CAD build for the part. Positions are in the model's coordinates, mm. A direction names the side the tool comes from. Round coordinates to 2 decimals unless told otherwise and drop trailing zeros. Write each loop counter-clockwise with the first axis right and the second up, starting at its lowest first coordinate (ties: lowest second). Pieces come first, ordered by that corner, then holes. Notation, with made-up numbers: (65.25, 74.25) -> (74.25, 74.25) arc R32 cw to (74.25, 109.25) -> close; hole circle Ø3 at (-1, 26). An arc over 180 degrees is marked (long way). Put each result on its own line as item: value. Start each with the question number.
1. Drill centre lines: line 1 (Z direction, x = 33.9, y = 0); line 2 (Y direction, x = 35.8, z = 16); line 3 (Y direction, x = 34.5, z = 37.5). Where is each one in solid material? Low to high. Write a range as from..to.
2. 3-axis set-ups, long thin cutter, end or side, ignore diameter. For faces 4 (the flat face through (36, 2, 20)), 5 (the cylindrical face through (39.82, 5.56, 40.66)), 6 (the cylindrical face through (35.637, -0.432, 71.197)), 7 (the flat face through (37, 14, 41)): which of +Z, -Z, +X, -X, +Y, -Y reach the whole face in a straight line?
3. Saw through at C-C on z = 41.2. List the corners of the cut face in (x, y).
4. Saw through at A-A on z = 8. List the corners of the cut face in (x, y).
5. Flat gauge pins, fed straight in: P1, Ø3.5, axis at x = 36, y = -10.5, coming from the +Z side; P2, Ø8, axis at y = -8, z = 41.2, coming from the +X side; P3, Ø17.5, axis at y = 10.5, z = 13.5, coming from the +X side; P4, Ø1.4, axis at y = 11, z = 16, coming from the +X side. Where does each tip first touch, or does it go through?
6. Pull direction X, two halves, no side cores. Call faces 1 (the cylindrical face through (36.608, -10.399, -4.437)), 2 (the flat face through (39.2, 7, 42)), 3 (the flat face through (35, 11, -9)): pulls with the +X half, pulls with the -X half, needs draft (parallel to the pull), parting line crosses it, or undercut.
7. Saw through at D-D on y = 22.5. List the corners of the cut face in (x, z), and give its area (3 significant figures).
8. Saw through at B-B on z = 22. List the corners of the cut face in (x, y), and give its area (3 significant figures).
from build123d import *

# Parameters (mm, degrees)
SKETCH_1_W          = 9
SKETCH_1_H          = 60
EXTRUDE_1_DEPTH     = 41.2
SKETCH_4_R          = 30
EXTRUDE_3_DEPTH     = 9
CUT_EXTRUDE_1_DEPTH = 72
SKETCH_5_R          = 15.7
CUT_EXTRUDE_2_DEPTH = 3
SKETCH_6_W          = 4
SKETCH_6_H          = 28
CUT_EXTRUDE_3_DEPTH = 3
SKETCH_7_W          = 3
SKETCH_7_H          = 4
CUT_EXTRUDE_4_DEPTH = 39.2
SKETCH_8_W          = 4
SKETCH_8_H          = 82.4
CUT_EXTRUDE_5_DEPTH = 25
SKETCH_9_R          = 2
EXTRUDE_4_DEPTH     = 9
SKETCH_10_R         = 0.8
CUT_EXTRUDE_6_DEPTH = 5
SKETCH_11_R         = 1
CUT_EXTRUDE_7_DEPTH = 1
SKETCH_12_R         = 2.5
CUT_EXTRUDE_9_DEPTH = 2


with BuildPart() as part:
    # 草图1 → 凸台-拉伸1 (new body)
    with BuildSketch(Plane.XY):
        with Locations((36.7, 0)):
            Rectangle(SKETCH_1_W, SKETCH_1_H)
    extrude(amount=EXTRUDE_1_DEPTH)

    # 草图4 → 凸台-拉伸3 (add)
    with BuildSketch(Plane.ZY.offset(-32.2)):
        with Locations((41.2, 0)):
            Circle(SKETCH_4_R)
    extrude(amount=-EXTRUDE_3_DEPTH)

    # 切除-拉伸1: read off the stored shape, not the designer's step
    # 切除-拉伸1 outline → 切除-拉伸1 (cut)
    with BuildSketch(Plane.XY):
        with BuildLine():
            Line((32.2, 30), (32.2, 25.702139989))
            ThreePointArc((32.2, 25.702139989), (38.884958532, 13.616166862), (41.2, 0))
            Line((41.2, 0), (41.2, 30))
            Line((41.2, 30), (32.2, 30))
        make_face()
        with BuildLine():
            Line((41.2, -30), (41.2, 0))
            ThreePointArc((41.2, 0), (38.884958532, -13.616166862), (32.2, -25.702139989))
            Line((32.2, -25.702139989), (32.2, -30))
            Line((32.2, -30), (41.2, -30))
        make_face()
    extrude(amount=CUT_EXTRUDE_1_DEPTH, mode=Mode.SUBTRACT)

    # 草图5 → 切除-拉伸2 (cut)
    with BuildSketch(Plane.ZY.offset(-32.2)):
        with Locations((41.2, 0)):
            Circle(SKETCH_5_R)
    extrude(amount=-CUT_EXTRUDE_2_DEPTH, mode=Mode.SUBTRACT)

    # 草图6 → 切除-拉伸3 (cut)
    with BuildSketch(Plane.ZY.offset(-35.2)):
        with Locations((41.2, 0)):
            Rectangle(SKETCH_6_W, SKETCH_6_H)
    extrude(amount=-CUT_EXTRUDE_3_DEPTH, mode=Mode.SUBTRACT)

    # 草图7 → 切除-拉伸4 (cut)
    with BuildSketch(Plane.XY.offset(39.2)):
        with Locations((36.7, 0)):
            Rectangle(SKETCH_7_W, SKETCH_7_H)
    extrude(amount=-CUT_EXTRUDE_4_DEPTH, mode=Mode.SUBTRACT)

    # 草图8 → 切除-拉伸5 (cut)
    with BuildSketch(Plane.XY):
        with Locations((39.2, 0)):
            Rectangle(SKETCH_8_W, SKETCH_8_H)
    extrude(amount=CUT_EXTRUDE_5_DEPTH, mode=Mode.SUBTRACT)

    # 草图9 → 凸台-拉伸4 (add)
    with BuildSketch(Plane.XY):
        with Locations((34.7, 11)):
            Circle(SKETCH_9_R)
        with Locations((34.7, -11)):
            Circle(SKETCH_9_R)
    extrude(amount=-EXTRUDE_4_DEPTH)

    # 草图10 → 切除-拉伸6 (cut)
    with BuildSketch(Plane(origin=(37.2, 0, 0), x_dir=(0, 0, -1), z_dir=(1, 0, 0))):
        with Locations((-16, -11)):
            Circle(SKETCH_10_R)
        with Locations((-8, -11)):
            Circle(SKETCH_10_R)
        with Locations((-16, 11)):
            Circle(SKETCH_10_R)
        with Locations((-8, 11)):
            Circle(SKETCH_10_R)
    extrude(amount=-CUT_EXTRUDE_6_DEPTH, mode=Mode.SUBTRACT)

    # 草图11 → 切除-拉伸7 (cut)
    with BuildSketch(Plane.ZY.offset(-38.2)):
        with Locations((41.2, 8)):
            Circle(SKETCH_11_R)
        with Locations((41.2, -8)):
            Circle(SKETCH_11_R)
    extrude(amount=-CUT_EXTRUDE_7_DEPTH, mode=Mode.SUBTRACT)

    # 草图12 → 切除-拉伸9 (cut)
    with BuildSketch(Plane.ZY.offset(-39.2)):
        with Locations((41.2, 8)):
            Circle(SKETCH_12_R)
        with Locations((41.2, -8)):
            Circle(SKETCH_12_R)
    extrude(amount=-CUT_EXTRUDE_9_DEPTH, mode=Mode.SUBTRACT)


solid = part.part
Return value:
1. line 1: z = 0..25.5, 56.9..71.2
1. line 2: y = -20.39..-11.8, -10.2..-2, 2..10.2, 11.8..20.39
1. line 3: y = -22.52..-15.26, 15.26..22.52
2. face 4: -Z
2. face 5: +X
2. face 6: +Z, +X, -X
2. face 7: -X
3. outline: (32.2, -25.7) arc R41.2 ccw to (39.84, -10.5) -> (39.2, -10.5) -> (39.2, -9) -> (38.2, -9) -> (38.2, -14) -> (35.2, -14) -> (35.2, -15.7) -> (32.2, -15.7) -> close; (32.2, 15.7) -> (35.2, 15.7) -> (35.2, 14) -> (38.2, 14) -> (38.2, 9) -> (39.2, 9) -> (39.2, 10.5) -> (39.84, 10.5) arc R41.2 ccw to (32.2, 25.7) -> close; (38.2, -7) -> (39.2, -7) -> (39.2, -5.5) -> (40.83, -5.5) arc R41.2 ccw to (40.83, 5.5) -> (39.2, 5.5) -> (39.2, 7) -> (38.2, 7) -> close
4. outline: (32.2, -25.7) arc R41.2 ccw to (37.2, -17.71) -> (37.2, -11.8) -> (32.2, -11.8) -> close; (32.2, -10.2) -> (37.2, -10.2) -> (37.2, -2) -> (35.2, -2) -> (35.2, 2) -> (37.2, 2) -> (37.2, 10.2) -> (32.2, 10.2) -> close; (32.2, 11.8) -> (37.2, 11.8) -> (37.2, 17.71) arc R41.2 ccw to (32.2, 25.7) -> close
5. P1: stops at z = 69.9
5. P2: stops at x = 41.01
5. P3: stops at x = 37.2
5. P4: passes through
6. face 1: parting line crosses it
6. face 2: pulls with the +X half
6. face 3: needs draft
7. outline: (32.2, 0) -> (34.51, 0) -> (34.51, 61.04) -> (32.2, 61.04) -> close
7. area: 141 mm^2
8. outline: (32.2, -25.7) arc R41.2 ccw to (37.2, -17.71) -> (37.2, -2) -> (35.2, -2) -> (35.2, 2) -> (37.2, 2) -> (37.2, 17.71) arc R41.2 ccw to (32.2, 25.7) -> close
8. area: 212 mm^2
